Geometry: final body of the model. Coordinates: model frame, mm. A direction names the side the tool comes from. Give positions to 0.01 mm unless a question says otherwise; leave off trailing zeros. Write each loop counter-clockwise with the first axis right and the second up, starting at its lowest first coordinate (ties: lowest second). Pieces come first, ordered by that corner, then holes. Notation, with made-up numbers: (-20, 37) -> (2, 37) arc R18 ccw to (2, 62) -> close; hole circle Ø1 at (1, 73). An arc over 180 degrees is marked (long way). Answer as a JSON object with one key per item and string values. Group by question number.
(1) Section query C-C on y = -39.5. Output: boundary loops of the cut face in (x, z).
(2) Contact query for flat-ended pins moving along their axis: pin 1 Ø8.5 at (x, z) = (-14.22, -32.38) entering from +Y; pin 2 Ø5 at (x, z) = (-14.22, 9.62) entering from -Y; pin 3 Ø1.5 at (x, y) = (-8, -23.5) entering from -Z; pin 4 Ø2 at (y, z) = (-19, 13.5) entering from +X. Output: stop coordinate, or through.
(3) Section query B-B on z = 10. Output: boundary loops of the cut face in (x, y).
(4) Material intervals for probe 1 along Z at (x, y) = (-14, -27); probe 2 along Z at (x, y) = (-15.5, -28); probe 3 along X at (y, z) = (-3, 20.5), sorted ascending.
(5) Section query A-A on y = -9. Output: boundary loops of the cut face in (x, z), plus the area to 3 significant figures.
(6) Section query D-D on x = -4. Output: boundary loops of the cut face in (y, z).
(7) Draft query along Z for faces 1 (the face through (-16.273, -20.713, -32.84)), 2 (the face through (-2.1, -12.2, 21.2)), 3 (the face through (8, -17, 23.615)). Return one class per face: +Z half, -Z half, draft (parallel to the pull), parting line (faces both ways), or undercut.
(8) Set-up query: faces 4 (the face through (-12, -41.5, -33)), 5 (the face through (12.9, -28.2, 21.2)), 6 (the face through (-1, -26, 18.615)). Return all of +Z, -Z, +X, -X, +Y, -Y with unobstructed straight access to the full face (end or side cutting, diameter ignored); none if empty.
from build123d import *

# Parameters (mm, degrees)
SKETCH1_W           = 25
SKETCH1_H           = 50
SKETCH1_R           = 3.4
BOSS_EXTRUDE1_DEPTH = 3
SKETCH2_W           = 50
SKETCH2_H           = 3
BOSS_EXTRUDE2_DEPTH = 8
SKETCH3_W           = 8
SKETCH3_H           = 50
BOSS_EXTRUDE3_DEPTH = 42
SKETCH4_R           = 2.65
CUT_EXTRUDE1_DEPTH  = 0.5
SKETCH5_R           = 5.802370205
CUT_EXTRUDE2_DEPTH  = 9
FILLET2_R           = 1
SKETCH6_R           = 12.6
BOSS_EXTRUDE4_DEPTH = 2
FILLET4_R           = 1
SKETCH8_R           = 1.589780168
SKETCH8_R_2         = 1.777428262
CUT_EXTRUDE3_DEPTH  = 10
SKETCH9_W           = 49.021678163
SKETCH9_H           = 20.976854622
CUT_EXTRUDE4_DEPTH  = 68.79439129
SKETCH11_R          = 2.1
CUT_EXTRUDE5_DEPTH  = 59.480168703
SKETCH14_R          = 2.6
CUT_EXTRUDE6_DEPTH  = 0.5
SKETCH15_W          = 8
SKETCH15_H          = 42
BOSS_EXTRUDE5_DEPTH = 10
SKETCH17_W          = 5
SKETCH17_H          = 42
BOSS_EXTRUDE6_DEPTH = 35
CUT_EXTRUDE7_DEPTH  = 5
SKETCH22_R          = 1.5
CUT_EXTRUDE8_DEPTH  = 5
CHAMFER1_SIZE       = 0.5


with BuildPart() as part:
    # Sketch1 → Boss-Extrude1 (new body)
    with BuildSketch(Plane(origin=(0, 0, 0), x_dir=(1, 0, 0), z_dir=(0, 1, 0))):
        with Locations((2.276951673, 11.384758364)):
            Rectangle(SKETCH1_W, SKETCH1_H)
        with Locations(Location((1.276951673, 11.384758364, 0), (0, 0, 270))):
            Circle(SKETCH1_R, mode=Mode.SUBTRACT)
    extrude(amount=BOSS_EXTRUDE1_DEPTH)

    # Sketch2 → Boss-Extrude2 (add)
    with BuildSketch(Plane.ZY.offset(10.223048327)):
        with Locations((-11.384758364, 1.5)):
            Rectangle(SKETCH2_W, SKETCH2_H)
    extrude(amount=BOSS_EXTRUDE2_DEPTH)

    # Sketch3 → Boss-Extrude3 (add)
    with BuildSketch(Plane.XZ):
        with Locations((-14.223048327, -11.384758364)):
            Rectangle(SKETCH3_W, SKETCH3_H)
    extrude(amount=BOSS_EXTRUDE3_DEPTH)

    # Sketch4 → Cut-Extrude1 (cut)
    with BuildSketch(Plane(origin=(0, 3, 0), x_dir=(1, 0, 0), z_dir=(0, 1, 0))):
        with Locations(Location((-14.223048327, 32.384758364, 0), (0, 0, 270))):
            Circle(SKETCH4_R)
        with Locations(Location((-14.223048327, -9.615241636, 0), (0, 0, 270))):
            Circle(SKETCH4_R)
    cut_extrude1 = extrude(amount=-CUT_EXTRUDE1_DEPTH, mode=Mode.SUBTRACT)

    # Mirror1: Cut-Extrude1 across plane
    add(cut_extrude1.mirror(Plane.ZX.offset(-19.5)), mode=Mode.SUBTRACT)

    # Sketch5 → Cut-Extrude2 (cut)
    with BuildSketch(Plane.ZY.offset(18.223048327)):
        with Locations((-11.836279124, -21)):
            Circle(SKETCH5_R)
    extrude(amount=-CUT_EXTRUDE2_DEPTH, mode=Mode.SUBTRACT)

    # Fillet2
    fillet2_edges = [part.edges().sort_by_distance(p)[0] for p in [
        (-10.223048327, -21, -17.638649329),
    ]]
    fillet(fillet2_edges, radius=FILLET2_R)

    # Mirror2: Cut-Extrude1 across plane
    add(cut_extrude1.mirror(Plane.ZY.offset(1.723048327)), mode=Mode.SUBTRACT)

    # Sketch6 → Boss-Extrude4 (add)
    with BuildSketch(Plane(origin=(0, 3, 0), x_dir=(1, 0, 0), z_dir=(0, 1, 0))):
        with BuildLine():
            Line((14.776951673, 5.825082115), (14.776951673, 16.944434614))
            ThreePointArc((14.776951673, 16.944434614), (-13.323048327, 11.384758364), (14.776951673, 5.825082115))
        make_face()
        with Locations(Location((1.276951673, 11.384758364, 0), (0, 0, 270))):
            Circle(SKETCH6_R, mode=Mode.SUBTRACT)
    extrude(amount=BOSS_EXTRUDE4_DEPTH)

    # Fillet4
    # the kernel refuses this fillet: 1 mm, written as the material it takes off along each edge
    with BuildSketch(Plane(origin=(14.776951673, 5, -3.325082115), x_dir=(0, -1, 0), z_dir=(0, 0, -1))) as fillet4_piece_1:
        with BuildLine():
            CenterArc((FILLET4_R, FILLET4_R), FILLET4_R, 180, 90)
            Line((0, FILLET4_R), (0, 0))
            Line((0, 0), (FILLET4_R, 0))
        make_face()
    extrude(amount=16.119352499, mode=Mode.SUBTRACT)

    # Sketch8 → Cut-Extrude3 (cut)
    with BuildSketch(Plane(origin=(0, 3, 0), x_dir=(1, 0, 0), z_dir=(0, 1, 0))):
        with Locations(Location((1.276951673, 19.884758364, 0), (0, 0, 270))):
            Circle(SKETCH8_R)
        with Locations(Location((1.276951673, 2.884758364, 0), (0, 0, 270))):
            Circle(SKETCH8_R_2)
    extrude(amount=-CUT_EXTRUDE3_DEPTH, mode=Mode.SUBTRACT)

    # Sketch9 → Cut-Extrude4 (cut, through all)
    with BuildSketch(Plane.XY.offset(13.615241636)):
        with Locations((-9.733887409, 10.488427311)):
            Rectangle(SKETCH9_W, SKETCH9_H)
    extrude(amount=-CUT_EXTRUDE4_DEPTH, mode=Mode.SUBTRACT)

    # Sketch11 → Cut-Extrude5 (cut, through all)
    with BuildSketch(Plane(origin=(0, 0, 0), x_dir=(1, 0, 0), z_dir=(0, 1, 0))):
        with Locations(Location((-14.223048327, 32.384758364, 0), (0, 0, 270))):
            Circle(SKETCH11_R)
    cut_extrude5 = extrude(amount=-CUT_EXTRUDE5_DEPTH, mode=Mode.SUBTRACT)

    # Mirror3: Cut-Extrude5 across plane
    add(cut_extrude5.mirror(Plane.XY.offset(-11.384758364)), mode=Mode.SUBTRACT)

    # Sketch14 → Cut-Extrude6 (cut)
    with BuildSketch(Plane(origin=(0, 0, 0), x_dir=(1, 0, 0), z_dir=(0, 1, 0))):
        with Locations(Location((-14.223048327, -9.615241636, 0), (0, 0, 270))):
            Circle(SKETCH14_R)
    cut_extrude6 = extrude(amount=-CUT_EXTRUDE6_DEPTH, mode=Mode.SUBTRACT)

    # Mirror4: Cut-Extrude6 across plane
    add(cut_extrude6.mirror(Plane.XY.offset(-11.384758364)), mode=Mode.SUBTRACT)

    # Sketch15 → Boss-Extrude5 (add)
    with BuildSketch(Plane.XY.offset(13.615241636)):
        with Locations((-14.223048327, -21)):
            Rectangle(SKETCH15_W, SKETCH15_H)
    extrude(amount=BOSS_EXTRUDE5_DEPTH)

    # Sketch17 → Boss-Extrude6 (add)
    with BuildSketch(Plane(origin=(-10.223048327, 0, 0), x_dir=(0, 0, -1), z_dir=(1, 0, 0))):
        with Locations((-21.115241636, -21)):
            Rectangle(SKETCH17_W, SKETCH17_H)
    extrude(amount=BOSS_EXTRUDE6_DEPTH)

    # Sketch21 → Cut-Extrude7 (cut)
    with BuildSketch(Plane.XY.offset(23.615241636)):
        Polygon((3.40621966, -21), (-10.223048327, -6.462114147), (-10.223048327, -35.537885853), align=None)
        Polygon((18.40621966, -5), (-8.852316315, -5), (4.776951673, -19.537885853), align=None)
        Polygon((19.776951673, -35.537885853), (19.776951673, -6.462114147), (6.147683685, -21), align=None)
        Polygon((4.776951673, -22.462114147), (-8.852316315, -37), (18.40621966, -37), align=None)
    extrude(amount=-CUT_EXTRUDE7_DEPTH, mode=Mode.SUBTRACT)

    # Sketch22 → Cut-Extrude8 (cut)
    with BuildSketch(Plane.XY.offset(23.615241636)):
        with Locations((22.276951673, -2.5)):
            Circle(SKETCH22_R)
        with Locations((22.276951673, -39.5)):
            Circle(SKETCH22_R)
        with Locations((4.776951673, -2.5)):
            Circle(SKETCH22_R)
    extrude(amount=-CUT_EXTRUDE8_DEPTH, mode=Mode.SUBTRACT)

    # Chamfer1
    chamfer1_edges = [part.edges().sort_by_distance(p)[0] for p in [
        (3.276951673, -2.5, 18.615241636),
        (20.776951673, -39.5, 18.615241636),
        (20.776951673, -2.5, 18.615241636),
    ]]
    chamfer(chamfer1_edges, length=CHAMFER1_SIZE)


solid = part.part
Answer list:
{
 "1": {"outline": "(-18.22, -36.38) -> (-10.22, -36.38) -> (-10.22, 18.62) -> (20.28, 18.62) -> (20.78, 19.12) -> (20.78, 23.62) -> (-18.22, 23.62) -> close; (23.78, 19.12) -> (24.28, 18.62) -> (24.78, 18.62) -> (24.78, 23.62) -> (23.78, 23.62) -> close; hole circle Ø4.2 at (-14.22, -32.38); hole circle Ø4.2 at (-14.22, 9.62)"},
 "2": {"pin 1": "y = 0", "pin 2": "y = -41.5", "pin 3": "through", "pin 4": "x = -10.22"},
 "3": {"outline": "(-18.22, -42) -> (-16.84, -42) -> (-16.84, -41.5) -> (-16.29, -41.5) -> (-16.29, -0.5) -> (-16.79, -0.5) -> (-16.79, 0) -> (-18.22, 0) -> close; (-12.16, -41.5) -> (-11.6, -41.5) -> (-11.6, -42) -> (-10.22, -42) -> (-10.22, 0) -> (-11.65, 0) -> (-11.65, -0.5) -> (-12.16, -0.5) -> close"},
 "4": {"probe 1": "-36.38 to -34.47, -30.3 to 7.53, 11.7 to 23.62", "probe 2": "-36.38 to -34.05, -30.72 to 7.95, 11.28 to 23.62", "probe 3": "-18.22 to 3.36, 6.19 to 20.86, 23.69 to 24.78"},
 "5": {"outline": "(-18.22, -36.38) -> (-10.22, -36.38) -> (-10.22, 23.62) -> (-18.22, 23.62) -> close; (-7.84, 18.62) -> (-5.1, 18.62) -> (-5.1, 23.62) -> (-7.84, 23.62) -> close; (14.66, 18.62) -> (17.4, 18.62) -> (17.4, 23.62) -> (14.66, 23.62) -> close; (19.78, 18.62) -> (24.78, 18.62) -> (24.78, 23.62) -> (19.78, 23.62) -> close; hole circle Ø4.2 at (-14.22, -32.38); hole circle Ø4.2 at (-14.22, 9.62)", "area": "505 mm2"},
 "6": {"outline": "(-42, 18.62) -> (-37, 18.62) -> (-37, 23.62) -> (-42, 23.62) -> close; (-31.82, 18.62) -> (-28.9, 18.62) -> (-28.9, 23.62) -> (-31.82, 23.62) -> close; (-13.1, 18.62) -> (-10.18, 18.62) -> (-10.18, 23.62) -> (-13.1, 23.62) -> close; (-5, 18.62) -> (0, 18.62) -> (0, 23.62) -> (-5, 23.62) -> close"},
 "7": {"face 1": "undercut", "face 2": "draft", "face 3": "+Z half"},
 "8": {"face 4": "-Y", "face 5": "+Z, -Z", "face 6": "-Z, +X, +Y, -Y"}
}
